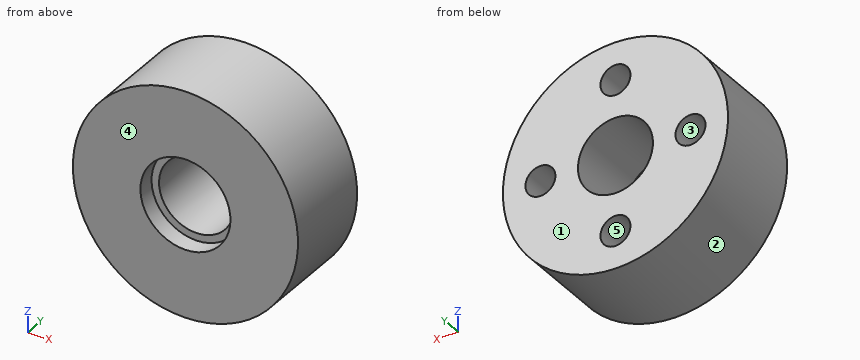
```python
from build123d import *

# Parameters (mm, degrees)
SKETCH1_R           = 30
BOSS_EXTRUDE1_DEPTH = 50
SKETCH2_R           = 75
BOSS_EXTRUDE2_DEPTH = 50
SKETCH3_R           = 25
SKETCH3_R_2         = 10
CUT_EXTRUDE1_DEPTH  = 50
BOSS_EXTRUDE4_START = 11.56865
SKETCH5_R           = 75
SKETCH5_R_2         = 30
BOSS_EXTRUDE4_DEPTH = 11.56865


with BuildPart() as part:
    # Sketch1 → Boss-Extrude1 (new body)
    with BuildSketch(Plane(origin=(0, 0, 0), x_dir=(1, 0, 0), z_dir=(0, 1, 0))):
        with Locations(Location((0, 0, 0), (0, 0, 270))):
            Circle(SKETCH1_R)
    extrude(amount=BOSS_EXTRUDE1_DEPTH)

    # Sketch2 → Boss-Extrude2 (add)
    with BuildSketch(Plane(origin=(0, 0, 0), x_dir=(-1, 0, 0), z_dir=(0, -1, 0))):
        with Locations(Location((0, 0, 0), (0, 0, 90))):
            Circle(SKETCH2_R)
    extrude(amount=-BOSS_EXTRUDE2_DEPTH)

    # Sketch3 → Cut-Extrude1 (cut)
    with BuildSketch(Plane(origin=(0, 50, 0), x_dir=(1, 0, 0), z_dir=(0, 1, 0))):
        with Locations(Location((0, 0, 0), (0, 0, 270))):
            Circle(SKETCH3_R)
        with Locations(Location((0, -50, 0), (0, 0, 270))):
            Circle(SKETCH3_R_2)
        with Locations(Location((50, 0, 0), (0, 0, 270))):
            Circle(SKETCH3_R_2)
        with Locations(Location((0, 50, 0), (0, 0, 270))):
            Circle(SKETCH3_R_2)
        with Locations(Location((-50, 0, 0), (0, 0, 270))):
            Circle(SKETCH3_R_2)
    extrude(amount=-CUT_EXTRUDE1_DEPTH, mode=Mode.SUBTRACT)

    # Sketch5 → Boss-Extrude4 (add)
    with BuildSketch(Plane(origin=(0, 0, 0), x_dir=(-1, 0, 0), z_dir=(0, -1, 0)).offset(BOSS_EXTRUDE4_START)):
        with Locations(Location((0, 0, 0), (0, 0, 90))):
            Circle(SKETCH5_R)
        with Locations(Location((0, 0, 0), (0, 0, 90))):
            Circle(SKETCH5_R_2, mode=Mode.SUBTRACT)
    extrude(amount=-BOSS_EXTRUDE4_DEPTH)


solid = part.part
```
Verification items for the finished model (mm, model axes). Face numbers are marked on the shaded views. A direction names the side the tool comes from. Coordinates: 2 decimals unless noted, no trailing zeros. Loops run counter-clockwise (first coordinate to the right, second up) from the corner with the lowest first, then second, coordinate; pieces in that order, holes last. Notation, with made-up numbers: (57, -22.5) - (107, -22.5) arc R16 ccw to (107, -5.5) - close; hole circle Ø2 at (-34.5, 10). An arc over 180 degrees is marked (long way). Put each result on its own line as item: value.
Item 1: Draft check along X on the marked faces 1, 2 and 3. Enter one of: pulls with the +X half, pulls with the -X half, needs draft (parallel to the pull), parting line crosses it, or undercut.
Conclusion:
face 1: needs draft
face 2: parting line crosses it
face 3: undercut
Item 2: Section check B-B (z = 0). Enter the section's corners in (x, y), then the cut area to 3 significant figures.
Conclusion:
outline: (-75, -11.57) - (-30, -11.57) - (-30, 0) - (-25, 0) - (-25, 50) - (-40, 50) - (-40, 0) - (-60, 0) - (-60, 50) - (-75, 50) - close; (25, 0) - (30, 0) - (30, -11.57) - (75, -11.57) - (75, 50) - (60, 50) - (60, 0) - (40, 0) - (40, 50) - (25, 50) - close
area: 4,040 mm2
Item 3: Set-up check for the marked faces 4 and 5: record each of +Z, -Z, +X, -X, +Y, -Y from which the full face is reachable in a straight line by a thin tool's end or side.
Conclusion:
face 4: +Z, -Z, +X, -X, -Y
face 5: +Y
Item 4: Section check D-D (z = 50). Enter the section's corners in (x, y).
Conclusion:
outline: (-55.9, -11.57) - (55.9, -11.57) - (55.9, 50) - (10, 50) - (10, 0) - (-10, 0) - (-10, 50) - (-55.9, 50) - close
Item 5: Section check C-C (y = 29.5). Enter the section's corners in (x, z).
Conclusion:
outline: circle Ø150 at (0, 0); hole circle Ø20 at (-50, 0); hole circle Ø50 at (0, 0); hole circle Ø20 at (0, -50); hole circle Ø20 at (0, 50); hole circle Ø20 at (50, 0)
Item 6: Gauge pin test, flat ends, axial feed: pin 1 Ø5 at (y, z) = (35.5, 48.5) entering from +X; pin 2 Ø1 at (y, z) = (2.5, 53) entering from +X; pin 3 Ø12 at (x, y) = (-28.5, 42) entering from -Z; pin 4 Ø22 at (x, z) = (-47.5, 3.5) entering from +Y. Record the tip position at first contact, or that the pin passes through.
Conclusion:
pin 1: stops at x = 59.24
pin 2: stops at x = 53.56
pin 3: stops at z = -71.55
pin 4: stops at y = 50
Item 7: Section check A-A (x = 0). Enter the section's corners in (y, z).
Conclusion:
outline: (-11.57, -75) - (50, -75) - (50, -60) - (0, -60) - (0, -40) - (50, -40) - (50, -25) - (0, -25) - (0, -30) - (-11.57, -30) - close; (-11.57, 30) - (0, 30) - (0, 25) - (50, 25) - (50, 40) - (0, 40) - (0, 60) - (50, 60) - (50, 75) - (-11.57, 75) - close
Item 8: Scan lines: line 1 along X through (y, z) = (38, 0); line 2 along X through (y, z) = (-2, 0); line 3 along Z through (x, y) = (-5.5, 23.5). Record each from-to range of solid material in increasing order.
Conclusion:
line 1: x = -75 to -60, -40 to -25, 25 to 40, 60 to 75
line 2: x = -75 to -30, 30 to 75
line 3: z = -74.8 to -58.35, -41.65 to -24.39, 24.39 to 41.65, 58.35 to 74.8
